Work out the finished part from the listing and answer in its coordinate system (mm). A direction names the side the tool comes from. Coordinates: 2 decimals unless noted, no trailing zeros. Write each loop counter-clockwise with the first axis right and the second up, starting at its lowest first coordinate (ties: lowest second). Pieces come first, ordered by that corner, then holes. Notation, with made-up numbers: (22.5, -20.75) - (69.5, -20.75) arc R15 cw to (69.5, 1.25) - close; hole circle Ø2 at (-10, 47.25). An arc over 180 degrees is marked (long way). Use one line per item in the form item = value. Start each with the question number.
Item 1: A cutting plane is placed at C-C (y = 35). Write down the section's boundary in (x, z), then the cut area to 3 significant figures.
Item 2: Determine the mould class of faces 1 (the cylindrical face through (-52.03, -71.79, 3.94)), 2 (the flat face through (-121.72, -76.69, 3.94)), 3 (the flat face through (-77, 1, 8)) for opening direction Y: released by +Y, released by -Y, zero draft, split by the parting line, or undercut.
Item 3: A cutting plane is placed at D-D (x = -94.5). Write down the section's boundary in (y, z).
Item 4: Consider probe 1 along Y at (x, z) = (-120, 3.75); probe 2 along Y at (x, z) = (-49.5, 6.75); probe 3 along Y at (x, z) = (-122, 6.75). Determine where each line is inside the solid, lowest interval first.
Item 5: A cutting plane is placed at A-A (x = -134). Write down the section's boundary in (y, z), then the cut area to 3 significant figures.
Item 6: For faces 4 (the flat face through (-126, 30, 4)), 5 (the flat face through (-34, -1, 4)), 6 (the flat face through (-110, 35, 4)), determine the directions among +Z, -Z, +X, -X, +Y, -Y from which every point of the face is accessible in a straight line to the end or side of a thin tool.
Item 7: Given pin 1 (4 mm diameter, centred on x = -130.5, z = 3, fed in from +Y); pin 2 (2.5 mm diameter, centred on y = -16, z = 2, fed in from -X); pin 3 (2.5 mm diameter, centred on x = -122, z = 6, fed in from -Y), each flat-ended and moving along its own axis, determine where each tip first touches the part or whether it passes through.
Item 8: A cutting plane is placed at B-B (z = 3). Give the number of separate pieces and of enclosed holes in the cut face, then the cut area to 3 significant figures.
Autodesk Inventor part; units mm, degrees
ref_plane "YZ Plane" through (0, 0, 0) normal (1, 0, 0) x (0, 1, 0)
ref_plane "XZ Plane" through (0, 0, 0) normal (0, 1, 0) x (-1, 0, 0)
ref_plane "XY Plane" through (0, 0, 0) normal (0, 0, 1) x (1, 0, 0)
sketch "Esquisse1" plane through (0, 0, 0) normal (0, 0, 1) x (1, 0, 0)
  line L0 (-44, 90) -> (-88, 90)
  line L1 (-102, -90) -> (-44, -90)
  line L2 (-34, -80) -> (-34, 80)
  line L3 (-88, 90) -> (-142, 63)
  line L4 (-102, -90) -> (-142, -63)
  line L5 (-44, 90) -> (-34, 80)
  line L6 (-44, -90) -> (-34, -80)
  line L7 (-80, 40) -> (-110, 40)
  line L8 (-110, -40) -> (-80, -40)
  line L9 (-80, -40) -> (-80, 40)
  line L10 (-142, 30) -> (-110, 30)
  line L11 (-110, -30) -> (-142, -30)
  line L12 (-142, 63) -> (-142, 30)
  line L13 (-142, -30) -> (-142, -63)
  line L14 (-110, 40) -> (-110, 30)
  line L15 (-110, -30) -> (-110, -40)
  line L16 (346.6566, 90) -> (-88, 90)
  point P0 (0, 0)
  point P1 (-34, 90)
  point P2 (-142, -90)
  point P3 (-142, 90)
  point P4 (-34, -90)
  dimension "d10" = 180
  dimension "d15" = 54
  dimension "d16" = 27
  dimension "d17" = 40
  dimension "d18" = 27
  dimension "d19" = 10
  dimension "d20" = 10
  dimension "d21" = 10
  dimension "d22" = 10
  dimension "d23" = 80
  dimension "d25" = 40
  dimension "d26" = 46
  dimension "d28" = 60
  dimension "d29" = 30
  dimension "d53" = 108
  dimension "d55" = 90
  dimension "d56" = 80
  dimension "d75" = 108
  dimension "d76" = 108
  dimension "d77" = 76
  dimension "d79" = 32
  dimension "d97" = 90
extrude "Plaque" add sketch "Esquisse1" along normal blind 8
sketch "Esquisse2" plane through (0, 0, 8) normal (0, 0, 1) x (1, 0, 0)
  line L0 (-80, 40) -> (-80, -40)
  line L1 (-80, -40) -> (-110, -40)
  line L2 (-110, 30) -> (-110, 40)
  line L3 (-110, 40) -> (-80, 40)
  line L4 (-88, 90) -> (-142, 63)
  line L5 (-142, 63) -> (-142, 30)
  line L6 (-142, 30) -> (-110, 30)
  line L7 (-110, -30) -> (-142, -30)
  line L8 (-142, -30) -> (-142, -63)
  line L9 (-142, -63) -> (-102, -90)
  line L10 (-102, -90) -> (-44, -90)
  line L11 (-44, -90) -> (-34, -80)
  line L12 (-34, -80) -> (-34, 80)
  line L13 (-34, 80) -> (-44, 90)
  line L14 (-44, 90) -> (-88, 90)
  circle A0 centre (-120, -35) radius 2.5
  circle A1 centre (-134, -35) radius 2.5
  circle A2 centre (-120, 35) radius 2.5
  circle A3 centre (-134, 35) radius 2.5
  line L15 (-110, -40) -> (-110, -30)
  dimension "d33" = 5
  dimension "d34" = 5
  dimension "d35" = 5
  dimension "d36" = 5
  dimension "d38" = 5
  dimension "d39" = 5
  dimension "d40" = 5
  dimension "d41" = 5
  dimension "d42" = 14
  dimension "d43" = 14
  dimension "d80" = 10
  dimension "d81" = 10
  dimension "d82" = 8
extrude "Extrusion2" cut sketch "Esquisse2" against normal up to next contours A0 | A1 | A2 | A3
sketch "Esquisse4" plane through (0, 0, 8) normal (0, 0, 1) x (1, 0, 0)
  circle A0 centre (-120, 35) radius 2.5
  circle A1 centre (-120, -35) radius 2.5
  circle A2 centre (-134, -35) radius 2.5
  circle A3 centre (-134, 35) radius 2.5
  line L0 (-88, 90) -> (-142, 63)
  line L1 (-142, 63) -> (-142, 30)
  line L2 (-142, 30) -> (-110, 30)
  line L3 (-110, 30) -> (-110, 40)
  line L4 (-110, 40) -> (-80, 40)
  line L5 (-80, 40) -> (-80, -40)
  line L6 (-80, -40) -> (-110, -40)
  line L7 (-110, -40) -> (-110, -30)
  line L8 (-110, -30) -> (-142, -30)
  line L9 (-142, -30) -> (-142, -63)
  line L10 (-142, -63) -> (-102, -90)
  line L11 (-102, -90) -> (-44, -90)
  line L12 (-44, -90) -> (-34, -80)
  line L13 (-34, -80) -> (-34, 80)
  line L14 (-34, 80) -> (-44, 90)
  line L15 (-44, 90) -> (-88, 90)
  line L16 (-126, 53.1115) -> (-84.2229, 74)
  line L17 (-84.2229, 74) -> (-50, 74)
  line L18 (-50, -74) -> (-97.1054, -74)
  line L19 (-97.1054, -74) -> (-126, -54.4961)
  point P0 (0, 0)
  dimension "d106" = 16
hole "Perçage3" at (-126, 53.1115, 8) at (-50, 74, 8) at (-50, -74, 8) at (-126, -54.4961, 8) direction (0, 0, -1) diameter 6 end through all
properties part number "Support_Roue"
Answer:
q1.outline = (-142, 0) - (-136.5, 0) - (-136.5, 8) - (-142, 8) - close; (-131.5, 0) - (-122.5, 0) - (-122.5, 8) - (-131.5, 8) - close; (-117.5, 0) - (-110, 0) - (-110, 8) - (-117.5, 8) - close; (-80, 0) - (-34, 0) - (-34, 8) - (-80, 8) - close
q1.area = 544 mm²
q2.face_1 = undercut
q2.face_2 = released by -Y
q2.face_3 = zero draft
q3.outline = (-90, 0) - (-40, 0) - (-40, 8) - (-90, 8) - close; (40, 0) - (86.75, 0) - (86.75, 8) - (40, 8) - close
q4.probe_1 = -77.85 to -37.5, -32.5 to -30, 30 to 32.5, 37.5 to 74
q4.probe_2 = -90 to -76.96, -71.04 to 71.04, 76.96 to 90
q4.probe_3 = -76.5 to -36.5, -33.5 to -30, 30 to 33.5, 36.5 to 73
q5.outline = (-68.4, 0) - (-37.5, 0) - (-37.5, 8) - (-68.4, 8) - close; (-32.5, 0) - (-30, 0) - (-30, 8) - (-32.5, 8) - close; (30, 0) - (32.5, 0) - (32.5, 8) - (30, 8) - close; (37.5, 0) - (67, 0) - (67, 8) - (37.5, 8) - close
q5.area = 523 mm²
q6.face_4 = +Z, -Z, -X
q6.face_5 = +Z, -Z, +X, +Y, -Y
q6.face_6 = +Z, -Z
q7.pin_1 = 69.75
q7.pin_2 = -80
q7.pin_3 = -77.34
q8.separate_pieces = 1
q8.enclosed_holes = 8
q8.area = 13,600 mm²
